Check sheet for the modelled part. Datum: model origin and axes. Units: mm. A direction names the side the tool comes from. Round coordinates to 2 decimals unless told otherwise and drop trailing zeros. Answer in a Markdown table with one row per item.
```python
from build123d import *

# Parameters (mm, degrees)
SKETCH1_R           = 12.427436065
BOSS_EXTRUDE1_DEPTH = 5
CUT_EXTRUDE1_DEPTH  = 6
SKETCH8_R           = 1.5


with BuildPart() as part:
    # Sketch1 → Boss-Extrude1 (new body)
    with BuildSketch(Plane(origin=(0, 0, 0), x_dir=(1, 0, 0), z_dir=(0, 1, 0))):
        with Locations((-0.572563935, 0)):
            Circle(SKETCH1_R)
        with BuildLine():
            ThreePointArc((-9.837575138, 1.742446029), (-9.678767906, 2.44), (-9.467522018, 3.123503075))
            ThreePointArc((-9.467522018, 3.123503075), (-7.221418603, 3.838718032), (-7.725075989, 6.141508127))
            ThreePointArc((-7.725075989, 6.141508127), (-7.238767906, 6.66620397), (-6.714072063, 7.152512053))
            ThreePointArc((-6.714072063, 7.152512053), (-4.411281968, 6.648854668), (-3.696067011, 8.894958082))
            ThreePointArc((-3.696067011, 8.894958082), (-3.012563935, 9.10620397), (-2.315009965, 9.265011203))
            ThreePointArc((-2.315009965, 9.265011203), (-0.572563935, 7.677436065), (1.169882094, 9.265011203))
            ThreePointArc((1.169882094, 9.265011203), (1.867436065, 9.10620397), (2.55093914, 8.894958082))
            ThreePointArc((2.55093914, 8.894958082), (3.266154097, 6.648854668), (5.568944192, 7.152512053))
            ThreePointArc((5.568944192, 7.152512053), (6.093640035, 6.66620397), (6.579948118, 6.141508127))
            ThreePointArc((6.579948118, 6.141508127), (6.076290732, 3.838718032), (8.322394147, 3.123503075))
            ThreePointArc((8.322394147, 3.123503075), (8.533640035, 2.44), (8.692447267, 1.742446029))
            ThreePointArc((8.692447267, 1.742446029), (7.104872129, 0), (8.692447267, -1.742446029))
            ThreePointArc((8.692447267, -1.742446029), (8.533640035, -2.44), (8.322394147, -3.123503075))
            ThreePointArc((8.322394147, -3.123503075), (6.076290732, -3.838718032), (6.579948118, -6.141508127))
            ThreePointArc((6.579948118, -6.141508127), (6.093640035, -6.66620397), (5.568944192, -7.152512053))
            ThreePointArc((5.568944192, -7.152512053), (3.266154097, -6.648854668), (2.55093914, -8.894958082))
            ThreePointArc((2.55093914, -8.894958082), (1.867436065, -9.10620397), (1.169882094, -9.265011203))
            ThreePointArc((1.169882094, -9.265011203), (-0.572563935, -7.677436065), (-2.315009965, -9.265011203))
            ThreePointArc((-2.315009965, -9.265011203), (-3.012563935, -9.10620397), (-3.696067011, -8.894958082))
            ThreePointArc((-3.696067011, -8.894958082), (-4.411281968, -6.648854668), (-6.714072063, -7.152512053))
            ThreePointArc((-6.714072063, -7.152512053), (-7.238767906, -6.66620397), (-7.725075989, -6.141508127))
            ThreePointArc((-7.725075989, -6.141508127), (-7.221418603, -3.838718032), (-9.467522018, -3.123503075))
            ThreePointArc((-9.467522018, -3.123503075), (-9.678767906, -2.44), (-9.837575138, -1.742446029))
            ThreePointArc((-9.837575138, -1.742446029), (-8.25, 0), (-9.837575138, 1.742446029))
        make_face(mode=Mode.SUBTRACT)
    extrude(amount=BOSS_EXTRUDE1_DEPTH)

    # Sketch7 → Cut-Extrude1 (cut, through all)
    with BuildSketch(Plane(origin=(0, 5, 0), x_dir=(1, 0, 0), z_dir=(0, 1, 0))):
        Polygon((13.300548716, 0), (-14.205268785, 0), (-13.392288958, -15.44944458), (9.438894535, -14.771961391), align=None)
    extrude(amount=-CUT_EXTRUDE1_DEPTH, mode=Mode.SUBTRACT)

    # Sketch8 → Cut-Revolve2 (revolve, cut)
    with BuildSketch(Plane.XY):
        with Locations((11.854872129, 2.5)):
            Circle(SKETCH8_R)
    revolve(axis=Axis((-0.572563935, 5, 0), (0, -1, 0)), mode=Mode.SUBTRACT)


solid = part.part
```
1. Section check B-B, the plane z = -8.25. Count the separate pieces of the cut face and the enclosed holes in it, and give its area (3 significant figures).
Found:
| item | result |
|---|---|
| separate pieces | 3 |
| enclosed holes | 0 |
| area | 66.3 mm2 |
2. Go/stop test with flat-tipped pins: pin 1 (2 mm diameter, centred on y = 1, z = -6, fed in from +X); pin 2 (3 mm diameter, centred on y = 4, z = -9, fed in from -X). Record where each tip stops, or that it passes through.
Found:
| item | result |
|---|---|
| pin 1 | stops at x = 10.8 |
| pin 2 | stops at x = -10.48 |
3. Access from +Z, -Z, +X, -X, +Y, -Y to the whole of each face (thin tool, end or side, straight path). Record for faces 5 (the face through (9, 3, 0)), 6 (the face through (8.53, 2.46, -2.45)).
Found:
| item | result |
|---|---|
| face 5 | +Z, +X, -X, +Y, -Y |
| face 6 | +Y, -Y |
4. Draft check along Z on faces 1 (the face through (6.06, 2.46, -3.87)), 2 (the face through (-10, 3, 0)), 3 (the face through (-1, 5, -9)), 4 (the face through (-0.299, 4.493, -12.424)). Enter one of: +Z half, -Z half, draft (parallel to the pull), parting line (faces both ways), or undercut.
Found:
| item | result |
|---|---|
| face 1 | undercut |
| face 2 | +Z half |
| face 3 | draft |
| face 4 | -Z half |
5. Scan lines: L1, parallel to X at y = 3.5, z = -8.75; L2, parallel to X at y = 2.9, z = -5; L3, parallel to X at y = 1.6, z = -8.25. Record each from-to range of solid material in increasing order.
Found:
| item | result |
|---|---|
| L1 | x = -7.74 to -3.64, -2.19 to 1.04, 2.49 to 6.59 |
| L2 | x = -10.35 to -7.01, 5.87 to 9.2 |
| L3 | x = -8.19 to -3.54, -1.87 to 0.72, 2.39 to 7.04 |
